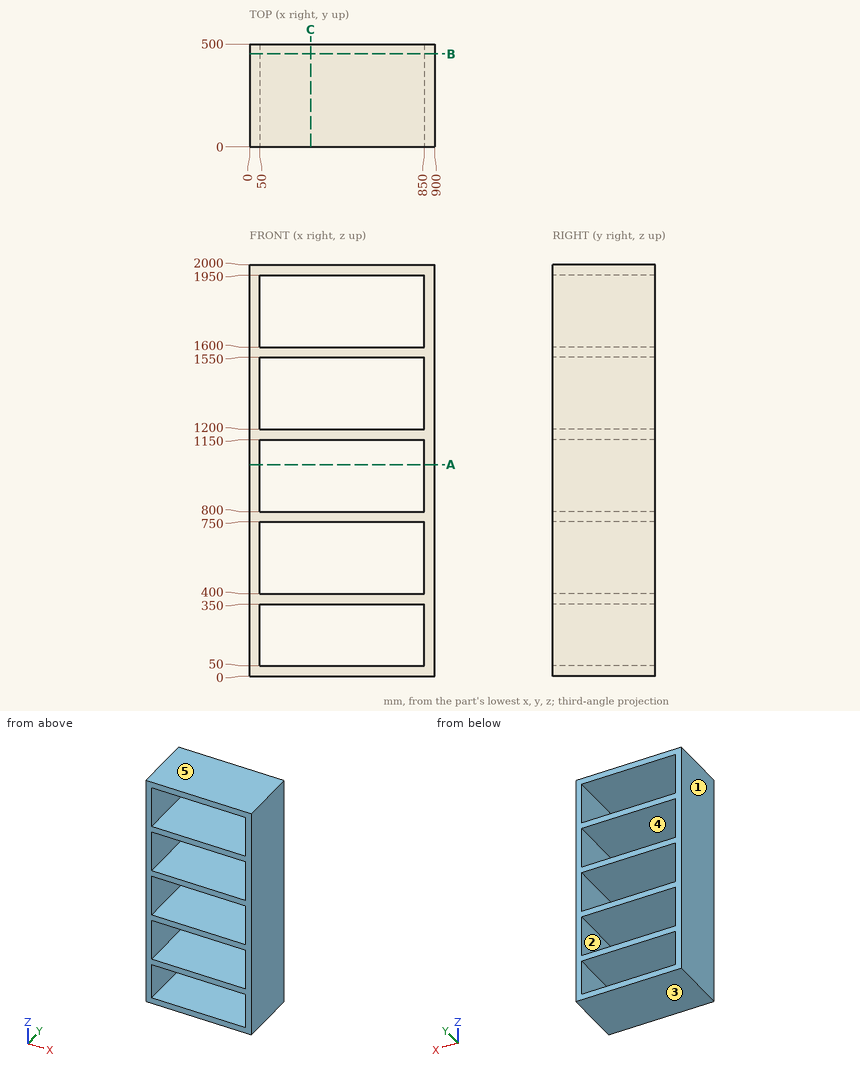
Can you work these out from the drawing? Everything is in mm from the part's minimum corner. A direction names the side the tool comes from. Coordinates: 2 decimals unless noted, no trailing zeros. Write each loop counter-clockwise with the first axis right and the second up, starting at its lowest first coordinate (ties: lowest second). Pieces come first, ordered by that corner, then holes. Notation, with made-up numbers: (36, 43) - (58, 43) arc R8 cw to (58, 56) - close; hole circle Ø9 at (41, 13.5). An arc over 180 degrees is marked (long way). One line per item, written item: value.
1) Suppose I cut it at C-C on x = 297.5. Write out the boundary of the cut face in (y, z).
Model answer:
outline: (0, 0) - (500, 0) - (500, 50) - (0, 50) - close; (0, 350) - (500, 350) - (500, 400) - (0, 400) - close; (0, 750) - (500, 750) - (500, 800) - (0, 800) - close; (0, 1150) - (500, 1150) - (500, 1200) - (0, 1200) - close; (0, 1550) - (500, 1550) - (500, 1600) - (0, 1600) - close; (0, 1950) - (500, 1950) - (500, 2000) - (0, 2000) - close
2) Suppose I cut it at A-A on z = 1028. Write out the boundary of the cut face in (x, y), and give its area (3 significant figures).
Model answer:
outline: (0, 0) - (50, 0) - (50, 500) - (0, 500) - close; (850, 0) - (900, 0) - (900, 500) - (850, 500) - close
area: 50,000 mm²
3) On a 3-axis mill with a long thin cutter (end or side, diameter ignored), from which of +Z, -Z, +X, -X, +Y, -Y can I reach the whole of each face in a straight line? I mean the marked faces 1 and 2. Say none if no direction works.
Model answer:
face 1: +Z, -Z, -X, +Y, -Y
face 2: +Y, -Y
4) I need wall thicknesses on line 1 along Z through (x, y) = (261, 193); line 2 along X through (y, z) = (302.5, 1090). Which ranges of each line are inside material? Lowest first, please.
Model answer:
line 1: z = 0 to 50, 350 to 400, 750 to 800, 1150 to 1200, 1550 to 1600, 1950 to 2000
line 2: x = 0 to 50, 850 to 900
5) Suppose I cut it at B-B on y = 451.5. Write out the boundary of the cut face in (x, z).
Model answer:
outline: (0, 0) - (900, 0) - (900, 2000) - (0, 2000) - close; hole (50, 50) - (850, 50) - (850, 350) - (50, 350) - close; hole (50, 400) - (850, 400) - (850, 750) - (50, 750) - close; hole (50, 800) - (850, 800) - (850, 1150) - (50, 1150) - close; hole (50, 1200) - (850, 1200) - (850, 1550) - (50, 1550) - close; hole (50, 1600) - (850, 1600) - (850, 1950) - (50, 1950) - close
6) We'd pull the mould along Z, two halves only. Please class the marked faces 3, 4 and 5: pulls with the +Z half, pulls with the -Z half, needs draft (parallel to the pull), parting line crosses it, or undercut.
Model answer:
face 3: pulls with the -Z half
face 4: undercut
face 5: pulls with the +Z half
